For this review, take the finished solid that the model builds, in its own axes (mm). A direction names the side the tool comes from. Coordinates: 2 decimals unless noted, no trailing zeros. Loops run counter-clockwise (first coordinate to the right, second up) from the corner with the lowest first, then second, coordinate; pieces in that order, holes last. Notation, with made-up numbers: M 79.25,38.25 L 97.25,38.25 A20 cw 97.25,70.25 Z; hole C 83.25,68 d3. An arc over 180 degrees is marked long. Put each result on its own line as item: value.
```python
from build123d import *

# Parameters (mm, degrees)
F1_DEPTH = 25.4


with BuildPart() as f1:
    # F0 (on Top) → F1 (new body)
    with BuildSketch(Plane.XY):
        Polygon((-31.274958, 46.557813), (-43.974958, 46.557813), (-43.974958, -34.902699), (-31.274958, -34.902699), (-31.274958, -3.152699), (-22.294702, 5.827557), (-31.274958, 14.807813), align=None)
        Polygon((-11.159787, 46.557813), (-31.274958, 14.807813), (-22.294702, 5.827557), (0, 40.495705), align=None)
        Polygon((-22.294702, 5.827557), (-31.274958, -3.152699), (-12.7, -34.902699), (0, -34.902699), align=None)
    extrude(amount=F1_DEPTH)


solid = f1.part
```
(1) Draft analysis for pull direction X (two halves, no side actions). For faces 6 (the flat face through (-5.502, 43.484, 12.522)), 7 (the flat face through (-21.077, 30.905, 12.522)), 8 (the flat face through (-38, -34.903, 13)), state which applies: +X half, -X half, draft (parallel to the pull), parting line (faces both ways), or undercut.
Determined:
face 6: +X half
face 7: undercut
face 8: draft
(2) Add section B-B (y = -18). Write out the cut boundary in (x, z), plus the area to 3 significant figures.
Determined:
outline: M -43.97,0 L -31.27,0 L -31.27,25.4 L -43.97,25.4 Z; M -22.59,0 L -9.25,0 L -9.25,25.4 L -22.59,25.4 Z
area: 661 mm^2
(3) Add section A-A (x = -20.5). Write out the cut boundary in (y, z).
Determined:
outline: M -21.57,0 L 2.55,0 L 2.55,25.4 L -21.57,25.4 Z; M 8.62,0 L 31.82,0 L 31.82,25.4 L 8.62,25.4 Z
(4) Wall thickness on line 1 along X through (y, z) = (16, 19); line 2 along X through (y, z) = (18, 15.25); line 3 along Y through (x, z) = (-15, 11.25): over which ranges is each line inside the solid? List them lowest first. Write a range as [from, to].
Determined:
line 1: x = [-43.97, -31.27], [-30.52, -15.75]
line 2: x = [-43.97, -31.27], [-29.25, -14.47]
line 3: y = [-30.97, -7.5], [17.17, 40.5]
(5) For pin 1 (8 mm diameter, centred on x = -27, z = 21.5, fed in from -Y); pin 2 (1 mm diameter, centred on x = -8.5, y = 23.5, fed in from -Z), all flat-tipped, find the tip position at first contact; note any pin that passes through.
Determined:
pin 1: stops at y = -17.3
pin 2: passes through
(6) Add section D-D (y = 14). Write out the cut boundary in (x, z), plus the area to 3 significant figures.
Determined:
outline: M -43.97,0 L -17.04,0 L -17.04,25.4 L -43.97,25.4 Z
area: 684 mm^2
(7) Tool access review of faces 1 (the flat face through (-31.275, -19, 13)), 2 (the flat face through (-43.975, 6, 13)), 3 (the flat face through (-31.275, 30, 13)), 4 (the flat face through (-6, -34.903, 13)), 5 (the flat face through (-11.303, 22.919, 12.522)): name each direction out of +Z, -Z, +X, -X, +Y, -Y from which nothing blocks a thin tool from reaching the whole face with its end or side.
Determined:
face 1: +Z, -Z, -Y
face 2: +Z, -Z, -X, +Y, -Y
face 3: +Z, -Z, +Y
face 4: +Z, -Z, +X, -X, -Y
face 5: +Z, -Z, +X
(8) Add section C-C (z = 11). Write out the cut boundary in (x, y), plus the area to 3 significant figures.
Determined:
outline: M -43.97,-34.9 L -31.27,-34.9 L -31.27,-3.15 L -12.7,-34.9 L 0,-34.9 L -22.29,5.83 L 0,40.5 L -11.16,46.56 L -31.27,14.81 L -31.27,46.56 L -43.97,46.56 Z
area: 2,090 mm^2
